The listing builds one solid part. Answer for the finished solid, in the listing's coordinates (mm). Coordinates: 2 decimals unless noted, no trailing zeros. Order: outer loops, then holes, each group sorted by start corner. A loop starts at its lowest first (then second) coordinate and runs counter-clockwise, first axis right, second up. Notation, with made-up numbers: M -28,2.5 L 25,2.5 A29 cw 25,31.5 Z; hole C 33.5,88.5 d8. An arc over 180 degrees is marked long. One line per item, written item: value. Start each with the question number.
Q1. Determine the mould class of faces 1 (the cylindrical face through (1.5, -4, 4)), 2 (the cylindrical face through (1.39, -4.23, 5.01)) for opening direction Z: pulls with the +Z half, pulls with the -Z half, needs draft (parallel to the pull), parting line crosses it, or undercut.
Q2. The part is cut by section B-B on x = 3. Give the vertices of the cut face in (y, z).
Q3. The part is cut by section A-A on z = 4. Give the vertices of the cut face in (x, y).
Q4. The part is cut by section C-C on y = -4. Give the vertices of the cut face in (x, z).
Q5. Straight lines are drawn through the part: line 1 along Z through (x, y) = (2.5, -2.45); line 2 along X through (y, z) = (-3.75, 4.05); line 3 along Z through (x, y) = (1.75, -5.75). For each, find the intervals that lie inside material, in ascending order. Write a range as [from, to].
Q6. The part is cut by section D-D on z = 2.7. Give the vertices of the cut face in (x, y).
```python
from build123d import *

# Parameters (mm, degrees)
CYLINDER001_R     = 1.5
CYLINDER001_DEPTH = 3
TUBE_R            = 1.5
TUBE_R_2          = 1
TUBE_DEPTH        = 7


with BuildPart() as cylinder001:
    # Cylinder001 → Cylinder001 (new body)
    with BuildSketch(Plane(origin=(1, 0, 4), x_dir=(0, 1, 0), z_dir=(1, 0, 0))):
        Circle(CYLINDER001_R)
    extrude(amount=CYLINDER001_DEPTH)


with BuildPart() as cut001:
    # Tube → Tube (new body)
    with BuildSketch(Plane(origin=(2.5, 0, 4), x_dir=(1, 0, 0), z_dir=(0, -1, 0))):
        Circle(TUBE_R)
        Circle(TUBE_R_2, mode=Mode.SUBTRACT)
    extrude(amount=TUBE_DEPTH)

    # Cut001: cut Cylinder001
    add(cylinder001.part, mode=Mode.SUBTRACT)


solid = cut001.part
```
Output:
1. face 1: undercut
1. face 2: parting line crosses it
2. outline: M -7,2.59 L -0.5,2.59 A1.5 cw -1.22,3.13 L -7,3.13 Z; M -7,4.87 L -1.22,4.87 A1.5 cw -0.5,5.41 L -7,5.41 Z
3. outline: M 1,-7 L 1.5,-7 L 1.5,-1.5 L 1,-1.5 Z; M 3.5,-7 L 4,-7 L 4,-1.5 L 3.5,-1.5 Z
4. outline: C 2.5,4 d3; hole C 2.5,4 d2
5. line 1: z = [2.5, 3], [5, 5.5]
5. line 2: x = [1, 1.5], [3.5, 4]
5. line 3: z = [2.7, 3.34], [4.66, 5.3]
6. outline: M 1.75,-7 L 3.25,-7 L 3.25,-0.75 L 1.75,-0.75 Z
